from build123d import *

# Parameters (mm, degrees)
SKETCH1_R               = 8.001
SKETCH1_R_2             = 6.477
BOSS_EXTRUDE1_DEPTH     = 245.11
CUT_EXTRUDE1_DEPTH      = 9.001
CUT_EXTRUDE1_DEPTH_BACK = 9.001


with BuildPart() as part:
    # Sketch1 → Boss-Extrude1 (new body)
    with BuildSketch(Plane.XY):
        Circle(SKETCH1_R)
        Circle(SKETCH1_R_2, mode=Mode.SUBTRACT)
    extrude(amount=BOSS_EXTRUDE1_DEPTH)

    # Sketch2 → Cut-Extrude1 (cut, two sides)
    with BuildSketch(Plane(origin=(0, 0, 0), x_dir=(0, 0, -1), z_dir=(1, 0, 0))) as cut_extrude1_sk:
        with BuildLine():
            Line((500.729314698, 3.175), (0, 3.175))
            Line((0, 3.175), (-27.94, 3.175))
            ThreePointArc((-27.94, 3.175), (-29.017630735, 2.728630735), (-29.464, 1.651))
            Line((-29.464, 1.651), (-29.464, -1.651))
            ThreePointArc((-29.464, -1.651), (-29.017630735, -2.728630735), (-27.94, -3.175))
            Line((-27.94, -3.175), (0, -3.175))
            Line((0, -3.175), (500.729314698, -3.175))
            Line((500.729314698, -3.175), (1502.187944094, -3.175))
            Line((1502.187944094, -3.175), (1502.187944094, 3.175))
            Line((1502.187944094, 3.175), (500.729314698, 3.175))
        make_face()
    extrude(amount=CUT_EXTRUDE1_DEPTH, mode=Mode.SUBTRACT)
    extrude(cut_extrude1_sk.sketch, amount=-CUT_EXTRUDE1_DEPTH_BACK, mode=Mode.SUBTRACT)


solid = part.part
Geometry: final body of the model. Coordinates: model frame, mm. Coordinates: 2 decimals unless noted, no trailing zeros. Loops run counter-clockwise (first coordinate to the right, second up) from the corner with the lowest first, then second, coordinate; pieces in that order, holes last. Notation, with made-up numbers: (15.5, 63) - (29.5, 63) arc R15 ccw to (29.5, 74) - close; hole circle Ø10 at (-17, 66). An arc over 180 degrees is marked (long way). Put each result on its own line as item: value. Start each with the question number.
Q1. Pin query (flat end, axial travel): pin 1 Ø1.4 at (x, y) = (7.5, 0.5) entering from -Z; pin 2 Ø1.4 at (x, z) = (6.5, 10) entering from -Y; pin 3 Ø2 at (y, z) = (4.5, 181) entering from +X. Return the tip coordinate at first contact, or that it passes through.
Q2. Cut plane A-A, the plane x = 0. Return loops of the section in (y, z).
Q3. Cut plane B-B, the plane z = 55.5. Return loops of the section in (x, y), and give its area (3 significant figures).
Q4. Line query: line 1 (X direction, y = -0.5, z = 70); line 2 (Y direction, x = 0.75, z = 100); line 3 (Y direction, x = -1.75, z = 182.5). Output: solid intervals per line, ascending.
Q5. Pull-direction query (X, two-part tool) for faces 1 (the flat face through (0, -7, 0)), 2 (the cylindrical face through (-8, 0, 121)), 3 (the cylindrical face through (-6.47, 0.28, 120.84)); classes: released by +X, released by -X, zero draft, split by the parting line, or undercut.
Filled sheet:
1. pin 1: z = 29.46
1. pin 2: y = -5.51
1. pin 3: x = 7.19
2. outline: (-8, 0) - (-6.48, 0) - (-6.48, 245.11) - (-8, 245.11) - close; (6.48, 0) - (8, 0) - (8, 245.11) - (6.48, 245.11) - close
3. outline: circle Ø16 at (0, 0); hole circle Ø12.95 at (0, 0)
3. area: 69.3 mm²
4. line 1: -7.99 to -6.46, 6.46 to 7.99
4. line 2: -7.97 to -6.43, 6.43 to 7.97
4. line 3: -7.81 to -6.24, 6.24 to 7.81
5. face 1: zero draft
5. face 2: split by the parting line
5. face 3: undercut
